Study the drawing (mm; zero at the part's minimum x, y, z) and answer. Coordinates: 2 decimals unless noted, no trailing zeros. Loops run counter-clockwise (first coordinate to the right, second up) from the corner with the lowest first, then second, coordinate; pieces in that order, holes last. Notation, with made-up numbers: (23, 43) - (79, 43) arc R9 ccw to (79, 59) - close; hole circle Ø1 at (-21.75, 12). An arc over 180 degrees is marked (long way). Put each result on its own line as item: value.
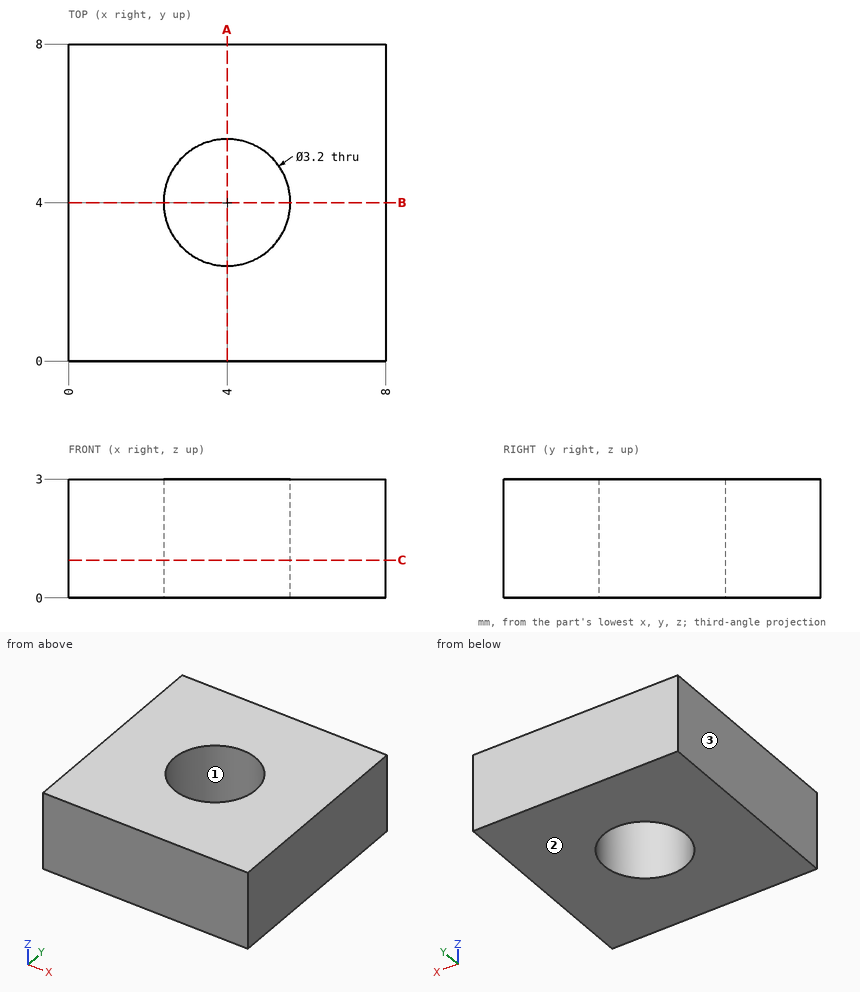
1) This flat-tipped pin is pushed along its axis until it touches: pin 1 (1.9 mm diameter, centred on x = 4, y = 4, fed in from -Z). Where does it stop, or does it pass through?
Found:
pin 1: passes through
2) The part is cut by section C-C (z = 0.95). Give the vertices of the cut face in (x, y).
Found:
outline: (0, 0) - (8, 0) - (8, 8) - (0, 8) - close; hole circle Ø3.2 at (4, 4)
3) The part is cut by section A-A (x = 4). Give the vertices of the cut face in (y, z).
Found:
outline: (0, 0) - (2.4, 0) - (2.4, 3) - (0, 3) - close; (5.6, 0) - (8, 0) - (8, 3) - (5.6, 3) - close
4) Straight lines are drawn through the part: L1, parallel to Y at x = 4, z = 1.05; L2, parallel to X at y = 4.5, z = 2.5; L3, parallel to X at y = 5.25, z = 1.4. For each, find the intervals that lie inside material, in ascending order. Write a range as [from, to].
Found:
L1: y = [0, 2.4], [5.6, 8]
L2: x = [0, 2.48], [5.52, 8]
L3: x = [0, 3], [5, 8]
5) For a pull along X with two mould halves and no side action, classify the marked faces 1, 2 and 3 as pulls with the +X half, pulls with the -X half, needs draft (parallel to the pull), parting line crosses it, or undercut.
Found:
face 1: undercut
face 2: needs draft
face 3: pulls with the -X half
